Source: CAD feature listing. Evaluate the final solid. Frame: model axes, mm. A direction names the side the tool comes from. Give positions to 0.01 mm unless a question says otherwise; leave off trailing zeros. Order: outer loops, then holes, each group sorted by start corner. A loop starts at its lowest first (then second) coordinate and runs counter-clockwise, first axis right, second up.
```python
from build123d import *

# Parameters (mm, degrees)
SKETCH1_W           = 150
SKETCH1_H           = 150
BOSS_EXTRUDE1_DEPTH = 10
SKETCH2_W           = 20
SKETCH2_H           = 150
BOSS_EXTRUDE2_DEPTH = 100
SKETCH3_R           = 7.9375
CUT_EXTRUDE1_DEPTH  = 201.561711201


with BuildPart() as part:
    # Sketch1 → Boss-Extrude1 (new body)
    with BuildSketch(Plane(origin=(0, 0, 0), x_dir=(1, 0, 0), z_dir=(0, 1, 0))):
        Rectangle(SKETCH1_W, SKETCH1_H)
    extrude(amount=BOSS_EXTRUDE1_DEPTH)

    # Sketch2 → Boss-Extrude2 (add)
    with BuildSketch(Plane(origin=(0, 10, 0), x_dir=(1, 0, 0), z_dir=(0, 1, 0))):
        with Locations((-65, 0)):
            Rectangle(SKETCH2_W, SKETCH2_H)
        with Locations((65, 0)):
            Rectangle(SKETCH2_W, SKETCH2_H)
    extrude(amount=BOSS_EXTRUDE2_DEPTH)

    # Sketch3 → Cut-Extrude1 (cut, through all)
    with BuildSketch(Plane(origin=(75, 0, 0), x_dir=(0, 0, -1), z_dir=(1, 0, 0))):
        with Locations((0, 65)):
            Circle(SKETCH3_R)
    extrude(amount=-CUT_EXTRUDE1_DEPTH, mode=Mode.SUBTRACT)


solid = part.part
```
1) Material intervals for L1, parallel to X at y = 71.5, z = 40; L2, parallel to Y at x = -70, z = 0; L3, parallel to Y at x = 18, z = 11.5, sorted ascending.
Report:
L1: x = -75 to -55, 55 to 75
L2: y = 0 to 57.06, 72.94 to 110
L3: y = 0 to 10
2) Section query B-B, the plane z = 0. Return the cut outline in (x, y), and give its area (4 significant figures).
Report:
outline: (-75, 0) - (75, 0) - (75, 57.06) - (55, 57.06) - (55, 10) - (-55, 10) - (-55, 57.06) - (-75, 57.06) - close; (-75, 72.94) - (-55, 72.94) - (-55, 110) - (-75, 110) - close; (55, 72.94) - (75, 72.94) - (75, 110) - (55, 110) - close
area: 4,865 mm2
3) Draft query along Y for faces 1 (the cylindrical face through (65.14, 57.25, 1.72)), 2 (the flat face through (-75, 54, 1)), 3 (the flat face through (-1, 10, -1)). Return one class per face: +Y half, -Y half, draft (parallel to the pull), parting line (faces both ways), or undercut.
Report:
face 1: undercut
face 2: draft
face 3: +Y half
4) Reachability of faces 4 (the flat face through (0, 2, 75)), 5 (the flat face through (-55, 48, 1)) from +Z, -Z, +X, -X, +Y, -Y: full face, straight path, thin tool, end or side. Return the list, or none.
Report:
face 4: +Z, +X, -X, +Y, -Y
face 5: +Z, -Z, +Y
5) Section query C-C, the plane y = 65. Return the cut outline in (x, z).
Report:
outline: (-75, -75) - (-55, -75) - (-55, -7.94) - (-75, -7.94) - close; (-75, 7.94) - (-55, 7.94) - (-55, 75) - (-75, 75) - close; (55, -75) - (75, -75) - (75, -7.94) - (55, -7.94) - close; (55, 7.94) - (75, 7.94) - (75, 75) - (55, 75) - close
6) Pin query (flat end, axial travel): pin 1 (3 mm diameter, centred on x = 36.5, z = -5, fed in from +Y). Return the tip coordinate at first contact, or that it passes through.
Report:
pin 1: stops at y = 10
7) Section query A-A, the plane y = 34.5. Return the cut outline in (x, z), and give its area (3 significant figures).
Report:
outline: (-75, -75) - (-55, -75) - (-55, 75) - (-75, 75) - close; (55, -75) - (75, -75) - (75, 75) - (55, 75) - close
area: 6,000 mm2
8) Section query D-D, the plane z = 56. Return the cut outline in (x, y), and give its area (3 significant figures).
Report:
outline: (-75, 0) - (75, 0) - (75, 110) - (55, 110) - (55, 10) - (-55, 10) - (-55, 110) - (-75, 110) - close
area: 5,500 mm2
